Read the model definition and answer for the solid it produces. Units are mm, in the model's axes. Face numbers are marked on the shaded views. Round coordinates to 2 decimals unless told otherwise and drop trailing zeros. Order: outer loops, then holes, each group sorted by start corner. A loop starts at its lowest first (then second) coordinate and runs counter-clockwise, first axis right, second up. Notation, with made-up numbers: (49.25, -38.5) - (64.25, -38.5) arc R14 ccw to (64.25, -19.5) - close; hole circle Ø1 at (77.25, 14.25). An arc over 180 degrees is marked (long way). Put each result on its own line as item: value. Start each with the question number.
Q1. For a pull along X with two mould halves and no side action, classify the marked faces 1, 2, 3 and 4 as pulls with the +X half, pulls with the -X half, needs draft (parallel to the pull), parting line crosses it, or undercut.
Q2. Section A-A on y = 7.5 is taken. Give the vertices of the cut face in (x, z), then the cut area to 3 significant figures.
Q3. Find the intervals of material crossed by line 1 along Z through (x, y) = (8.5, 5); line 2 along X through (y, z) = (6.25, 1.5); line 3 along Z through (x, y) = (-18.5, 9), in increasing order. Write a range as from..to.
Q4. Each of these flat-tipped pins is pushed along its axis until it touches: pin 1 Ø12 at (x, z) = (-1, 10) entering from +Y; pin 2 Ø5 at (x, y) = (-18.13, 5) entering from +Z; pin 3 Ø16 at (x, z) = (0, 0) entering from +Y; pin 4 Ø1 at (x, y) = (-12.5, 5.5) entering from +Z. Where does it stop, or does it pass through?
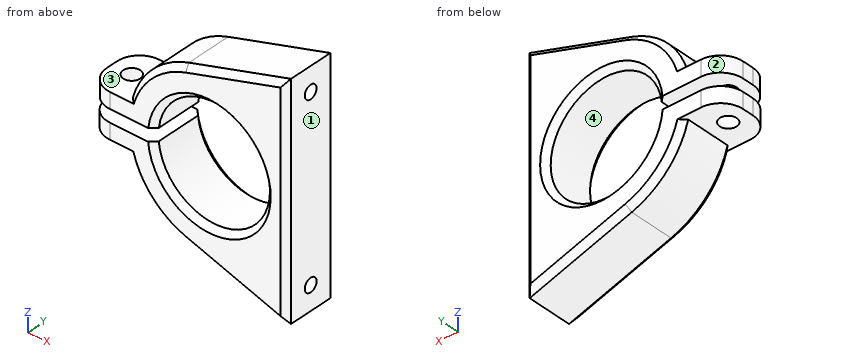
Autodesk Inventor part; units mm, degrees
ref_plane "YZ Plane" through (0, 0, 0) normal (1, 0, 0) x (0, 1, 0)
ref_plane "XZ Plane" through (0, 0, 0) normal (0, 1, 0) x (-1, 0, 0)
ref_plane "XY Plane" through (0, 0, 0) normal (0, 0, 1) x (1, 0, 0)
sketch "Эскиз1" plane through (0, 0, 0) normal (0, 1, 0) x (-1, 0, 0)
  arc A0 (9.8249, 1.217) -> (9.8505, -0.9889) centre (0, 0) ccw
  line L0 (-13.6311, 20) -> (-13.6311, -20)
  line L1 (-13.6311, 20) -> (4.492, 14.3116)
  line L2 (-13.6311, -20) -> (4.492, -14.3116)
  line L3 (9.8249, 1.217) -> (16.2051, 1.217)
  line L4 (13.6718, -0.9889) -> (9.8505, -0.9889)
  arc A1 (4.492, -14.3116) -> (14.5136, -3.7889) centre (0, 0) ccw
  arc A2 (14.4521, 4.017) -> (4.492, 14.3116) centre (0, 0) ccw
  line L5 (9.8505, -0.9889) -> (21.6521, -0.9889)
  line L6 (21.6521, -0.9889) -> (21.6521, -3.7889)
  line L7 (21.6521, -3.7889) -> (14.5136, -3.7889)
  line L8 (9.8249, 1.217) -> (21.6265, 1.217)
  line L9 (21.6265, 1.217) -> (21.6265, 4.017)
  line L10 (21.6265, 4.017) -> (14.4521, 4.017)
  point P0 (15, 0)
  dimension "d0" = 19.8
  dimension "d5" = 2.8
  dimension "d6" = 2.8
  dimension "d32" = 15
  dimension "d33" = 40
extrude "Выдавливание1" add sketch "Эскиз1" along normal blind 10
fillet "Сопряжение1" radius 4 4 edges at (-21.6265, 10, 2.617) (-21.6521, 10, -2.3889) (-21.6265, 0, 2.617) (-21.6521, 0, -2.3889)
sketch "Эскиз3" plane through (-14.4521, 0, 4.017) normal (0, 0, 1) x (1, 0, 0)
  arc A0 (-7.1744, 4) -> (-3.1744, 0) centre (-3.1744, 4) ccw
  line L0 (-3.1744, 0) -> (0, 0)
  line L1 (0, 0) -> (0, 10)
  line L2 (-3.1744, 10) -> (0, 10)
  arc A1 (-3.1744, 10) -> (-7.1744, 6) centre (-3.1744, 6) ccw
  line L3 (-7.1744, 4) -> (-7.1744, 6)
  line L4 (-7.1744, 5) -> (-3.6744, 5) construction
  point P0 (14.4521, 0)
  dimension "d20" = 3.5
hole "Отверстие2" at (-18.1265, 5, 4.017) direction (0, 0, -1) diameter 3 depth 8 tip angle 118
chamfer "Фаска1" distance 1 angle 45 12 edges at (9.8993, 10, -0.1148) (9.8993, 0, -0.1148) (4.5696, 10, 17.1558) (13.6311, 10, 0) (4.5696, 10, -17.1558) (-10.8621, 10, -10.3448) (-10.7803, 10, 10.43) (4.5696, 0, 17.1558) (13.6311, 0, 0) (4.5696, 0, -17.1558) (-10.8621, 0, -10.3448) (-10.7803, 0, 10.43)
sketch "Эскиз5" plane through (13.6311, 1, -20) normal (1, 0, 0) x (0, 0, -1)
  line L0 (-40, 0) -> (-40, 8) construction
  line L1 (0, 0) -> (0, 8) construction
  line L2 (-35.75, 4) -> (-40, 4) construction
  line L3 (-4.25, 4) -> (0, 4) construction
  point P0 (-20, -1)
  point P1 (-37.875, 4)
  dimension "d34" = 31.5
hole "Отверстие3" at (13.6311, 5, 15.75) at (13.6311, 5, -15.75) direction (-1, 0, 0) diameter 2.4 depth 8 tip angle 118
properties part number "VoiceMount"
Findings:
1. face 1: pulls with the +X half
1. face 2: pulls with the -X half
1. face 3: needs draft
1. face 4: undercut
2. outline: (-21.36, -3.79) - (-14.51, -3.79) arc R15 ccw to (-4.49, -14.31) - (13.63, -20) - (13.63, 20) - (-4.49, 14.31) arc R15 ccw to (-14.45, 4.02) - (-21.33, 4.02) - (-21.33, 1.22) - (-9.82, 1.22) arc R9.9 cw (long way) to (-9.85, -0.99) - (-21.36, -0.99) - close
2. area: 560 mm2
3. line 1: -18.39..-16.95, -14.55..-5.08, 5.08..14.55, 16.95..18.39
3. line 2: -21.62..-18.96, -17.3..-9.79, 9.79..13.63
3. line 3: -3.79..-0.99, 1.22..4.02
4. pin 1: y = 10
4. pin 2: z = 4.02
4. pin 3: through
4. pin 4: z = 9
